from build123d import *

# Parameters (mm, degrees)
SKETCH2_R           = 35
BOSS_EXTRUDE1_DEPTH = 3


with BuildPart() as part:
    # Sketch1 → Revolve-Thin1 (revolve)
    with BuildSketch(Plane.XY):
        Polygon((-80, 45), (-80, 35), (0, 35), (0, 30), (3, 30), (3, 38), (-77, 38), (-77, 45), align=None)
    revolve(axis=Axis((0, 0, 0), (-1, 0, 0)))

    # Sketch2 → Boss-Extrude1 (add)
    with BuildSketch(Plane.ZY.offset(80)):
        Circle(SKETCH2_R)
    extrude(amount=-BOSS_EXTRUDE1_DEPTH)


solid = part.part
Geometry check sheet. Reference: the model listing, model coordinates, mm. A direction names the side the tool comes from. Give positions to 0.01 mm unless a question says otherwise; leave off trailing zeros. Order: outer loops, then holes, each group sorted by start corner. A loop starts at its lowest first (then second) coordinate and runs counter-clockwise, first axis right, second up. Notation, with made-up numbers: (25.25, 5) - (84.25, 5) arc R17 ccw to (84.25, 18) - close; hole circle Ø2 at (-35, 59). An arc over 180 degrees is marked (long way). Answer as a JSON object with one key per item and string values.
(1) Tool access check on faces 4 (the flat face through (-77, 37, 10)), 5 (the flat face through (0, 26, -16)), 6 (the flat face through (-80, 1, -1)). Record the directions out of +Z, -Z, +X, -X, +Y, -Y that give a thin tool (end or side, any length) a straight path to the whole face; none if there is none.
Report:
{"face 4": "+X", "face 5": "none", "face 6": "+Z, -Z, -X, +Y, -Y"}
(2) Material ranges on line 1 (Z direction, x = -37, y = 0); line 2 (X direction, y = -16.5, z = -26.5), recorded low to high.
Report:
{"line 1": "-38 to -35, 35 to 38", "line 2": "-80 to -77, 0 to 3"}
(3) Draft check along Y on faces 1 (the flat face through (3, -28, -11.4)), 2 (the cylindrical face through (-37.56, 17.535, 33.713)), 3 (the cylindrical face through (1.52, -29.97, -1.32)). Enter one of: released by +Y, released by -Y, zero draft, split by the parting line, or undercut.
Report:
{"face 1": "zero draft", "face 2": "split by the parting line", "face 3": "undercut"}
(4) Cross-section at A-A (z = 0). Record the cut outline in (x, y).
Report:
{"outline": "(-80, -45) - (-77, -45) - (-77, -38) - (3, -38) - (3, -30) - (0, -30) - (0, -35) - (-77, -35) - (-77, 35) - (0, 35) - (0, 30) - (3, 30) - (3, 38) - (-77, 38) - (-77, 45) - (-80, 45) - close"}
(5) Cross-section at C-C (z = -31.5). Record the cut outline in (x, y), then the cut area to 3 significant figures.
Report:
{"outline": "(-80, -32.14) - (-77, -32.14) - (-77, -21.25) - (3, -21.25) - (3, 21.25) - (-77, 21.25) - (-77, 32.14) - (-80, 32.14) - close; hole (-77, -15.26) - (0, -15.26) - (0, 15.26) - (-77, 15.26) - close", "area": "1,240 mm^2"}
(6) Depth check by flat-ended pin: pin 1 Ø1 at (x, z) = (-29.5, -7.5) entering from -Y; pin 2 Ø5 at (y, z) = (18.5, -17.5) entering from +X; pin 3 Ø1 at (x, y) = (-36, 17) entering from +Z. Enter the tip coordinate at first touch or a pass-through.
Report:
{"pin 1": "y = -37.35", "pin 2": "x = -77", "pin 3": "z = 34.23"}
(7) Cross-section at D-D (x = -6). Record the cut outline in (y, z), then the cut area to 3 significant figures.
Report:
{"outline": "circle Ø76 at (0, 0); hole circle Ø70 at (0, 0)", "area": "688 mm^2"}
